Design review of the part built by this model. Coordinates are the model's own, in mm. A direction names the side the tool comes from. Round coordinates to 2 decimals unless told otherwise and drop trailing zeros. Loops run counter-clockwise (first coordinate to the right, second up) from the corner with the lowest first, then second, coordinate; pieces in that order, holes last. Notation, with made-up numbers: (18, -15) -> (37, -15) arc R22 cw to (37, 6) -> close; hole circle Ø9 at (63, -22). An arc over 180 degrees is marked (long way). Use a Markdown table: item, result. Add a question column.
from build123d import *

# Parameters (mm, degrees)
SKETCH_1_W          = 34
SKETCH_1_H          = 17
SKETCH_1_W_2        = 24
SKETCH_1_H_2        = 13
EXTRUDE_1_DEPTH     = 1.5
SKETCH_4_R          = 1
EXTRUDE_4_DEPTH     = 1
EXTRUDE_4_TAPER     = 43
SKETCH_3_W          = 34
SKETCH_3_H          = 2
EXTRUDE_5_DEPTH     = 7
SKETCH_5_W          = 1.698300115
SKETCH_5_H          = 2
SKETCH_5_W_2        = 29
EXTRUDE_6_DEPTH     = 15.5
CUT_EXTRUDE_1_REACH = 7
SKETCH_6_W          = 8
SKETCH_6_H          = 13
EXTRUDE_7_DEPTH     = 12
SKETCH_10_W         = 24
SKETCH_10_H         = 29.92364145
SKETCH_10_W_2       = 22.5
SKETCH_10_H_2       = 13
EXTRUDE_8_DEPTH     = 3
SKETCH_11_W         = 46
SKETCH_11_H         = 29.92364145
EXTRUDE_9_DEPTH     = 3
SKETCH_12_W         = 16.749756905
SKETCH_12_H         = 24.683929902
SKETCH_12_W_2       = 2.349687525
SKETCH_12_H_2       = 24.562319206
EXTRUDE_10_DEPTH    = 5.5
EXTRUDE_START       = -3.202635
EXTRUDE_11_DEPTH    = 3.202635
CUT_EXTRUDE_2_REACH = 26
SKETCH_14_R         = 2.5


with BuildPart() as part:
    # 草图1 → 凸台-拉伸1 (new body)
    with BuildSketch(Plane.XY):
        with Locations((-12, 6.5)):
            Rectangle(SKETCH_1_W, SKETCH_1_H)
        with Locations((-12, 6.5)):
            Rectangle(SKETCH_1_W_2, SKETCH_1_H_2, mode=Mode.SUBTRACT)
    extrude(amount=EXTRUDE_1_DEPTH)

    # 草图4 → 凸台-拉伸4 (add)
    with BuildSketch(Plane.XY):
        with Locations((2.6, 10)):
            Circle(SKETCH_4_R)
        with Locations((2.6, 3)):
            Circle(SKETCH_4_R)
        with Locations((-26.6, 10)):
            Circle(SKETCH_4_R)
        with Locations((-26.6, 3)):
            Circle(SKETCH_4_R)
    extrude(amount=-EXTRUDE_4_DEPTH, taper=EXTRUDE_4_TAPER)

    # 草图3 → 凸台-拉伸5 (add)
    with BuildSketch(Plane(origin=(0, 0, 0), x_dir=(-1, 0, 0), z_dir=(0, 0, -1))):
        with Locations((12, -1)):
            Rectangle(SKETCH_3_W, SKETCH_3_H)
        with Locations((12, 14)):
            Rectangle(SKETCH_3_W, SKETCH_3_H)
    extrude(amount=EXTRUDE_5_DEPTH)

    # 草图5 → 凸台-拉伸6 (add)
    with BuildSketch(Plane(origin=(0, 0, -7), x_dir=(-1, 0, 0), z_dir=(0, 0, -1))):
        with Locations((-0.849150058, -1)):
            Rectangle(SKETCH_5_W, SKETCH_5_H)
        with Locations((14.5, -1)):
            Rectangle(SKETCH_5_W_2, SKETCH_5_H)
        Polygon((0, 15), (-1.698300115, 15), (-1.698300115, 0), (0, 0), (0, 13), align=None)
        with Locations((14.5, 14)):
            Rectangle(SKETCH_5_W_2, SKETCH_5_H)
    extrude(amount=EXTRUDE_6_DEPTH)

    # 草图6 → 切除-拉伸1 (cut, up to next)
    with BuildSketch(Plane.ZY, mode=Mode.PRIVATE) as cut_extrude_1_sk1:
        with Locations((-18.5, 6.5)):
            Rectangle(SKETCH_6_W, SKETCH_6_H)
    cut_extrude_1_tool1 = extrude(cut_extrude_1_sk1.sketch, amount=-CUT_EXTRUDE_1_REACH, mode=Mode.PRIVATE) & part.part
    add(cut_extrude_1_tool1.solids().sort_by_distance((0, 6.5, -18.5))[0], mode=Mode.SUBTRACT)

    # 草图9 → 凸台-拉伸7 (add)
    with BuildSketch(Plane.ZY.offset(29)):
        Polygon((-22.5, 15), (1.5, 15), (1.5, -2), (-22.5, -2), (-22.5, 0), (0, 0), (0, 13), (-22.5, 13), align=None)
    extrude(amount=EXTRUDE_7_DEPTH)

    # 草图10 → 凸台-拉伸8 (add)
    with BuildSketch(Plane.ZY.offset(41)):
        with Locations((-10.5, -16.961820725)):
            Rectangle(SKETCH_10_W, SKETCH_10_H)
        with Locations((-11.25, 6.5)):
            Rectangle(SKETCH_10_W_2, SKETCH_10_H_2)
        Polygon((1.5, 15), (-22.5, 15), (-22.5, 13), (0, 13), (0, 0), (-22.5, 0), (-22.5, -2), (1.5, -2), align=None)
    extrude(amount=-EXTRUDE_8_DEPTH)

    # 草图11 → 凸台-拉伸9 (add)
    with BuildSketch(Plane.XY.offset(1.5)):
        with Locations((-18, -16.961820725)):
            Rectangle(SKETCH_11_W, SKETCH_11_H)
    extrude(amount=-EXTRUDE_9_DEPTH)

    # 草图12 → 凸台-拉伸10 (add)
    with BuildSketch(Plane(origin=(0, 0, -1.5), x_dir=(-1, 0, 0), z_dir=(0, 0, -1))):
        Polygon((-5, -2), (-5, -31.92364145), (16.5, -31.92364145), (16.5, -28.721006537), (16.5, -4.158687331), (16.5, -2), align=None)
        with Locations((5.65486472, -16.500652282)):
            Rectangle(SKETCH_12_W, SKETCH_12_H, mode=Mode.SUBTRACT)
        Polygon((16.5, -28.721006537), (16.5, -31.92364145), (38, -31.92364145), (38, -28.721006537), (35.650312475, -28.721006537), align=None)
        with Locations((36.825156237, -16.439846934)):
            Rectangle(SKETCH_12_W_2, SKETCH_12_H_2)
        Polygon((38, -2), (16.5, -2), (16.5, -4.158687331), (35.650312475, -4.158687331), (38, -4.158687331), align=None)
    extrude(amount=EXTRUDE_10_DEPTH)

    # 草图13 → 凸台-拉伸11 (add)
    with BuildSketch(Plane.XZ.offset(31.92364145).offset(EXTRUDE_START)):
        Polygon((-38, -22.5), (-22.5, -7), (-38, -7), align=None)
    extrude(amount=EXTRUDE_11_DEPTH)

    # 草图14 → 切除-拉伸2 (cut, up to next)
    with BuildSketch(Plane.XY.offset(1.5), mode=Mode.PRIVATE) as cut_extrude_2_sk1:
        with Locations((-6.493645673, -23.522660126)):
            Circle(SKETCH_14_R)
    cut_extrude_2_tool1 = extrude(cut_extrude_2_sk1.sketch, amount=-CUT_EXTRUDE_2_REACH, mode=Mode.PRIVATE) & part.part
    add(cut_extrude_2_tool1.solids().sort_by_distance((-6.493646, -23.52266, 1.5))[0], mode=Mode.SUBTRACT)


solid = part.part
1. For faces 1 (the face through (-38, 7, -11)), 2 (the face through (-18, -2, -15)), 3 (the face through (0, 6, -11)), 4 (the face through (-18, 15, -11)), 5 (the face through (2, 7, 0)), list the 3-axis set-ups (+Z, -Z, +X, -X, +Y, -Y) from which the entire face can be reached by the end or side of a thin tool; tool diameter is ignored.
2. Consider section A-A on z = -10.5. State the section outline as (x, y) points, plus the area to 3 significant figures.
3. Mouldability with a two-part tool opening along Y and no side actions: class faces 6 (the face through (1.698, 6, -11)), 7 (the face through (-31, 6, 0)), 8 (the face through (-23, -31.924, -5)) as +Y half, -Y half, draft (parallel to the pull), parting line (faces both ways), or undercut.
4. Consider section B-B on y = 1. State the section outline as (x, z) points.
5. To check wall thickness, follow probe 1 along Y at (x, z) = (-33.5, -4); probe 2 along Y at (x, z) = (2.5, -2.75); probe 3 along Y at (x, z) = (1.5, -20.25). State the ranges of each line that lie inside material, in increasing order. Write a range as from..to.
6. Consider section D-D on x = -29.5. State the section outline as (y, z) points, plus the area to 3 significant figures.
7. Consider section C-C on x = -15.5. State the section outline as (y, z) points.
8. Insertion check: P1, Ø0.5, axis at x = 0.5, y = 4.5, coming from the -Z side; P2, Ø12, axis at x = -6, z = -9, coming from the -Y side; P3, Ø6.5, axis at x = -33.5, y = 3.5, coming from the -Z side; P4, Ø9.5, axis at x = -19.5, y = -16.5, coming from the -Z side. Each pin has a flat end and moves straight along its axis. Give the tip position at first contact, or say it passes through.
Verdict:
| question | item | result |
|---|---|---|
| 1 | face 1 | -Z |
| 1 | face 2 | -Z, +X |
| 1 | face 3 | +Z, -Z |
| 1 | face 4 | +Z, -Z, +X, -X, +Y |
| 1 | face 5 | none |
| 2 | outline | (-41, -31.92) -> (-26, -31.92) -> (-26, -28.72) -> (-38, -28.72) -> (-38, -2) -> (1.7, -2) -> (1.7, 15) -> (-41, 15) -> close; hole (-38, 0) -> (0, 0) -> (0, 13) -> (-38, 13) -> close |
| 2 | area | 360 mm² |
| 3 | face 6 | draft |
| 3 | face 7 | undercut |
| 3 | face 8 | -Y half |
| 4 | outline | (-41, -22.5) -> (-38, -22.5) -> (-38, 0) -> (-24, 0) -> (-24, 1.5) -> (-41, 1.5) -> close; (0, -14.5) -> (1.7, -14.5) -> (1.7, -7) -> (0, -7) -> close; (0, 0) -> (5, 0) -> (5, 1.5) -> (0, 1.5) -> close |
| 5 | probe 1 | y = -31.92..-28.72, -4.16..0, 13..15 |
| 5 | probe 2 | y = -31.92..-28.84, -4.16..0, 13..15 |
| 5 | probe 3 | y = -2..0, 13..15 |
| 6 | outline | (-31.92, -14) -> (-28.72, -14) -> (-28.72, -1.5) -> (-4.16, -1.5) -> (-4.16, -7) -> (-2, -7) -> (-2, -22.5) -> (0, -22.5) -> (0, 0) -> (13, 0) -> (13, -22.5) -> (15, -22.5) -> (15, 1.5) -> (-31.92, 1.5) -> close |
| 6 | area | 257 mm² |
| 7 | outline | (-31.92, -7) -> (-2, -7) -> (-2, -22.5) -> (0, -22.5) -> (0, 1.5) -> (-31.92, 1.5) -> close; (13, -22.5) -> (15, -22.5) -> (15, 1.5) -> (13, 1.5) -> close |
| 8 | P1 | stops at z = -14.5 |
| 8 | P2 | stops at y = -31.92 |
| 8 | P3 | stops at z = 0 |
| 8 | P4 | stops at z = -7 |
